Design review of the part built by this model. Coordinates are the model's own, in mm. Face numbers are marked on the shaded views. A direction names the side the tool comes from. Round coordinates to 2 decimals unless told otherwise and drop trailing zeros. Write each loop counter-clockwise with the first axis right and the second up, starting at its lowest first coordinate (ties: lowest second). Pieces come first, ordered by that corner, then holes. Notation, with made-up numbers: (26, -38.5) -> (58, -38.5) arc R4 cw to (58, -33.5) -> close; hole circle Ø11 at (47, 20.25). An arc over 180 degrees is marked (long way). Write item = value, one per line. Start each with the question number.
Item 1: Add section C-C, the plane z = -3.15. State the section outline as (x, y) points, then the cut area to 3 significant figures.
Item 2: Add section A-A, the plane y = 0.2. State the section outline as (x, z) points (3 decimals), then the cut area to 3 significant figures.
Item 3: Mouldability with a two-part tool opening along X and no side actions: class the marked faces 3, 4 and 5 as released by +X, released by -X, zero draft, split by the parting line, or undercut.
Item 4: Machinability: for the marked faces 1 and 2, which of the approach directions +Z, -Z, +X, -X, +Y, -Y give a long, thin tool a straight path to every point of the face, cutting with its end or side? Answer none if there is none.
Item 5: To check wall thickness, follow L1, parallel to X at y = 1.4, z = -0.4 (3 decimals); L2, parallel to Z at x = 6.75, y = 0.95; L3, parallel to X at y = 0.3, z = -2.8. State the ranges of each line that lie inside material, in increasing order.
Item 6: Add section B-B, the plane x = 5.25. State the section outline as (y, z) points.
Item 7: For pin 1 Ø1 at (x, y) = (4, 1) entering from +Z, flat-tipped, find the tip position at first contact; note if it passes through.
from build123d import *

# Parameters (mm, degrees)
BOSS_EXTRUDE1_DEPTH = 2.25
SKETCH2_W           = 4
SKETCH2_H           = 2
CUT_EXTRUDE1_DEPTH  = 0.5


with BuildPart() as part:
    # Sketch1 → Boss-Extrude1 (new body)
    with BuildSketch(Plane(origin=(0, 0, 0), x_dir=(1, 0, 0), z_dir=(0, 1, 0))):
        Polygon((0, 0), (7.25, 0), (7.25, 0.5), (6.5, 0.5), (6.5, 3.5), (0.75, 3.5), (0.75, 0.5), (0, 0.5), align=None)
    extrude(amount=BOSS_EXTRUDE1_DEPTH)

    # Sketch2 → Cut-Extrude1 (cut)
    with BuildSketch(Plane.XY):
        with Locations((3.625, 1)):
            Rectangle(SKETCH2_W, SKETCH2_H)
    extrude(amount=-CUT_EXTRUDE1_DEPTH, mode=Mode.SUBTRACT)


solid = part.part
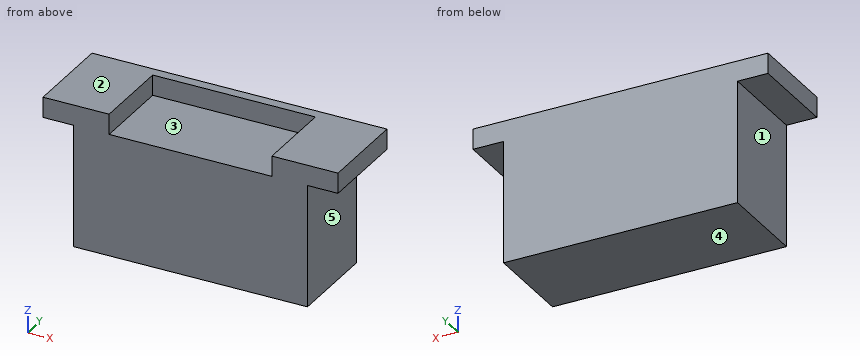
Result set:
q1.outline = (0.75, 0) -> (6.5, 0) -> (6.5, 2.25) -> (0.75, 2.25) -> close
q1.area = 12.9 mm²
q2.outline = (0, -0.5) -> (0.75, -0.5) -> (0.75, -3.5) -> (6.5, -3.5) -> (6.5, -0.5) -> (7.25, -0.5) -> (7.25, 0) -> (5.625, 0) -> (5.625, -0.5) -> (1.625, -0.5) -> (1.625, 0) -> (0, 0) -> close
q2.area = 18.9 mm²
q3.face_3 = undercut
q3.face_4 = zero draft
q3.face_5 = released by +X
q4.face_1 = -Z, -X, +Y, -Y
q4.face_2 = +Z, +X, -X, +Y, -Y
q5.L1 = 0 to 1.625, 5.625 to 7.25
q5.L2 = -0.5 to 0
q5.L3 = 0.75 to 6.5
q6.outline = (0, -3.5) -> (2.25, -3.5) -> (2.25, 0) -> (2, 0) -> (2, -0.5) -> (0, -0.5) -> close
q7.pin_1 = -0.5
